```python
from build123d import *

# Parameters (mm, degrees)
BOSS_EXTRUDE1_DEPTH = 4
SKETCH2_OUTSIDE_W   = 29.082
SKETCH2_OUTSIDE_H   = 30.606
SKETCH2_OUTSIDE_R   = 5.014305997
CUT_EXTRUDE1_DEPTH  = 4
CUT_EXTRUDE1_DRAFT  = -60
SKETCH3_OUTSIDE_W   = 29.082
SKETCH3_OUTSIDE_H   = 30.606
SKETCH3_OUTSIDE_R   = 5.014305997
CUT_EXTRUDE2_DEPTH  = 4
CUT_EXTRUDE2_DRAFT  = -60
SKETCH4_R           = 3
BOSS_EXTRUDE3_DEPTH = 3


with BuildPart() as part:
    # Sketch1 → Boss-Extrude1 (new body)
    with BuildSketch(Plane(origin=(0, 0, 0), x_dir=(1, 0, 0), z_dir=(0, 1, 0))):
        Polygon((5, 2.919649438), (-0.028490583, 5.789951738), (-5.028490583, 2.8703023), (-5, -2.919649438), (0.028490583, -5.789951738), (5.028490583, -2.8703023), align=None)
    extrude(amount=BOSS_EXTRUDE1_DEPTH)


with BuildPart() as cut_extrude1_tool:
    # Sketch2 outside → Cut-Extrude1 (with draft: the straight prism first)
    with BuildSketch(Plane(origin=(0, 4, 0), x_dir=(1, 0, 0), z_dir=(0, 1, 0))):
        Rectangle(SKETCH2_OUTSIDE_W, SKETCH2_OUTSIDE_H)
        Circle(SKETCH2_OUTSIDE_R, mode=Mode.SUBTRACT)
    extrude(amount=-CUT_EXTRUDE1_DEPTH)
    # Cut-Extrude1: the draft: its side faces are tilted about the plane it starts from
    cut_extrude1_sides = [cut_extrude1_tool.faces().sort_by_distance(p)[0] for p in [
        (0, 2, 15.303),
        (14.541, 2, 0),
        (0, 2, -15.303),
        (-14.541, 2, 0),
        (-5.014305997, 2, 0),
    ]]
    draft(cut_extrude1_sides, Plane(origin=(0, 4, 0), x_dir=(1, 0, 0), z_dir=(0, 1, 0)), CUT_EXTRUDE1_DRAFT)


with BuildPart() as part_1:
    add(part.part)

    # Cut-Extrude1: cut by cut_extrude1_tool
    add(cut_extrude1_tool.part, mode=Mode.SUBTRACT)


with BuildPart() as cut_extrude2_tool:
    # Sketch3 outside → Cut-Extrude2 (with draft: the straight prism first)
    with BuildSketch(Plane.XZ):
        Rectangle(SKETCH3_OUTSIDE_W, SKETCH3_OUTSIDE_H)
        Circle(SKETCH3_OUTSIDE_R, mode=Mode.SUBTRACT)
    extrude(amount=-CUT_EXTRUDE2_DEPTH)
    # Cut-Extrude2: the draft: its side faces are tilted about the plane it starts from
    cut_extrude2_sides = [cut_extrude2_tool.faces().sort_by_distance(p)[0] for p in [
        (0, 2, -15.303),
        (14.541, 2, 0),
        (0, 2, 15.303),
        (-14.541, 2, 0),
        (-5.014305997, 2, 0),
    ]]
    draft(cut_extrude2_sides, Plane.XZ, CUT_EXTRUDE2_DRAFT)


with BuildPart() as part_2:
    add(part_1.part)

    # Cut-Extrude2: cut by cut_extrude2_tool
    add(cut_extrude2_tool.part, mode=Mode.SUBTRACT)

    # Sketch4 → Boss-Extrude3 (add)
    with BuildSketch(Plane(origin=(0, 4, 0), x_dir=(1, 0, 0), z_dir=(0, 1, 0))):
        with Locations(Location((0, 0, 0), (0, 0, 270))):
            Circle(SKETCH4_R)
    extrude(amount=BOSS_EXTRUDE3_DEPTH)


solid = part_2.part
```
Geometry check sheet. Reference: the model listing, model coordinates, mm. A direction names the side the tool comes from. Round coordinates to 2 decimals unless told otherwise and drop trailing zeros. Order: outer loops, then holes, each group sorted by start corner. A loop starts at its lowest first (then second) coordinate and runs counter-clockwise, first axis right, second up. Notation, with made-up numbers: (8.5, 21.5) - (49.5, 21.5) arc R21 ccw to (49.5, 42.5) - close; hole circle Ø8 at (-17.75, 31). An arc over 180 degrees is marked (long way). Use a Markdown table: item, result. Add a question column.
1) Set-up check for faces 1 (the cylindrical face through (0.9, 5.48, 2.86)), 2 (the conical face through (0.013, 3.893, 5.199)): record each of +Z, -Z, +X, -X, +Y, -Y from which the full face is reachable in a straight line by a thin tool's end or side.
2) Section check C-C (y = 5.25). Record the cut outline in (x, z), then the cut area to 3 significant figures.
3) Section check A-A (y = 1). Record the cut outline in (x, z).
4) Thickness scan on line 1 along Y through (x, z) = (0, 3.75); line 2 along X through (y, z) = (2.75, -2.25); line 3 along X through (y, z) = (4.25, -2). Record the ranges inside material, lowest first.
5) Section check B-B (y = 3.75). Record the cut outline in (x, z).
6) Gauge pin test, flat ends, axial feed: P1, Ø1.5, axis at x = 0, z = 3.5, coming from the +Y side; P2, Ø4, axis at y = 3, z = 0, coming from the -X side; P3, Ø1.5, axis at x = -4, z = -1, coming from the +Y side; P4, Ø2, axis at y = 2.5, z = 0.5, coming from the +X side. Record the tip position at first contact, or that the pin passes through.
Established:
| question | item | result |
|---|---|---|
| 1 | face 1 | +Y |
| 1 | face 2 | +Z, +Y |
| 2 | outline | circle Ø6 at (0, 0) |
| 2 | area | 28.3 mm2 |
| 3 | outline | (-5.03, -2.87) - (-0.03, -5.79) - (5, -2.92) - (5.03, 2.87) - (0.03, 5.79) - (-5, 2.92) - close |
| 4 | line 1 | 0 to 4 |
| 4 | line 2 | -5.03 to 5 |
| 4 | line 3 | -2.24 to 2.24 |
| 5 | outline | (-5.02, -2.1) arc R5.45 ccw to (-4.37, -3.26) - (-0.69, -5.4) arc R5.45 ccw to (0.64, -5.41) - (4.33, -3.3) arc R5.45 ccw to (5, -2.15) - (5.02, 2.1) arc R5.45 ccw to (4.37, 3.26) - (0.69, 5.4) arc R5.45 ccw to (-0.64, 5.41) - (-4.33, 3.3) arc R5.45 ccw to (-5, 2.15) - close |
| 6 | P1 | y = 7 |
| 6 | P2 | x = -5.02 |
| 6 | P3 | y = 4 |
| 6 | P4 | x = 5.02 |
